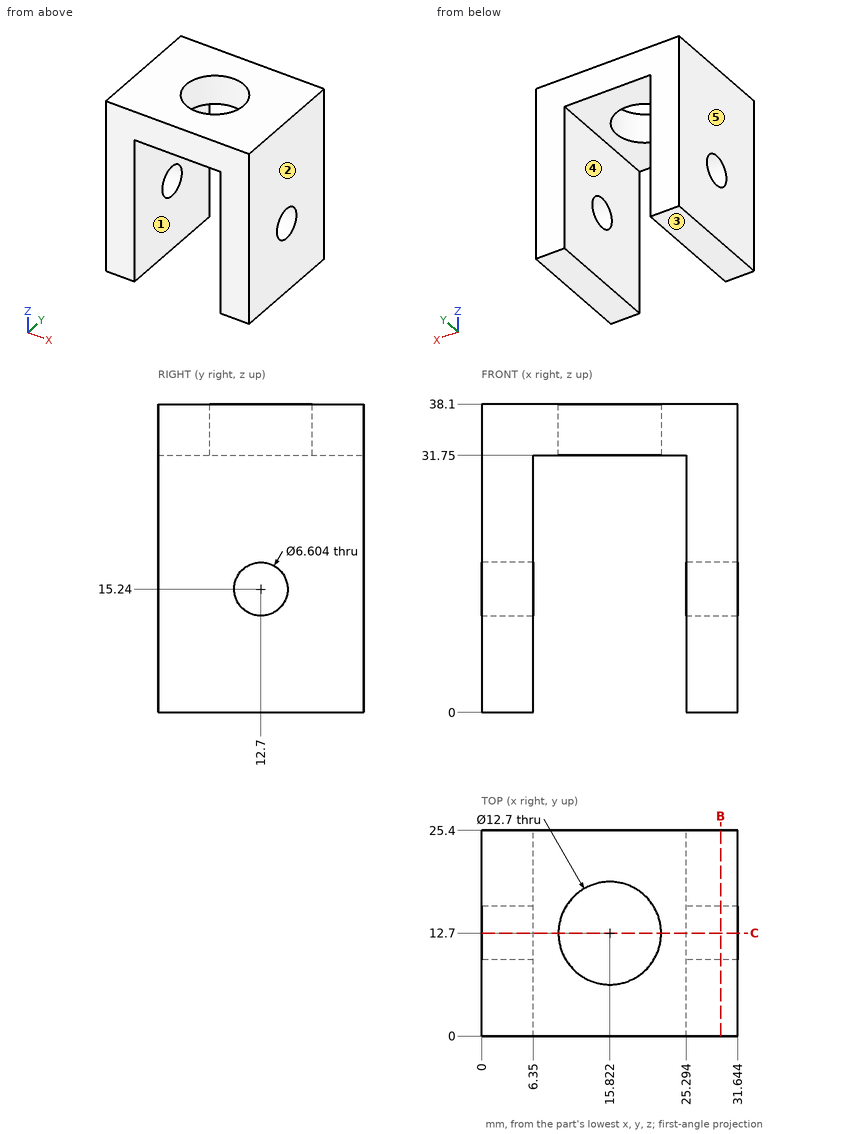
Geometry: see drawing. Coordinates: mm, zero at the bounding-box minimum. A direction names the side the tool comes from. Coordinates: 2 decimals unless noted, no trailing zeros. Loops run counter-clockwise (first coordinate to the right, second up) from the corner with the lowest first, then second, coordinate; pieces in that order, holes last. Notation, with made-up numbers: (62, -2.5) - (92, -2.5) arc R22 ccw to (92, 11.5) - close; hole circle Ø7 at (73.5, 81.5). An arc over 180 degrees is marked (long way). Answer in a Markdown table with one row per item.
(1) Material intervals for L1, parallel to Y at x = 27.5, z = 15; L2, parallel to Z at x = 10, y = 2.25; L3, parallel to X at y = 17.5, z = 36 (1 decimal), sorted ascending. Write a range as from..to.
Model answer:
| item | result |
|---|---|
| L1 | y = 0..9.41, 15.99..25.4 |
| L2 | z = 31.75..38.1 |
| L3 | x = 0..11.7, 20..31.6 |
(2) Cut plane C-C on y = 12.7. Count the separate pieces of the cut face and the enclosed holes in it.
Model answer:
| item | result |
|---|---|
| separate pieces | 4 |
| enclosed holes | 0 |
(3) Set-up query: the marked faces 1 and 2. Return all of +Z, -Z, +X, -X, +Y, -Y with unobstructed straight access to the full face (end or side cutting, diameter ignored); none if empty.
Model answer:
| item | result |
|---|---|
| face 1 | -Z, +Y, -Y |
| face 2 | +Z, -Z, +X, +Y, -Y |
(4) Mould query, pull axis X, two halves, no side actions, for the marked faces 3, 4 and 5. Classes: pulls with the +X half, pulls with the -X half, needs draft (parallel to the pull), parting line crosses it, or undercut.
Model answer:
| item | result |
|---|---|
| face 3 | needs draft |
| face 4 | undercut |
| face 5 | pulls with the -X half |
(5) Pin query (flat end, axial travel): P1, Ø14.5, axis at x = 15.82, y = 12.7, coming from the -Z side. Return the tip coordinate at first contact, or that it passes through.
Model answer:
| item | result |
|---|---|
| P1 | stops at z = 31.75 |
(6) Cut plane B-B on x = 29.5. Output: boundary loops of the cut face in (y, z).
Model answer:
| item | result |
|---|---|
| outline | (0, 0) - (25.4, 0) - (25.4, 38.1) - (0, 38.1) - close; hole circle Ø6.6 at (12.7, 15.24) |
